```python
from build123d import *

# Parameters (mm, degrees)
F0_R     = 88.9
F1_DEPTH = 50.8
F2_R     = 60.325
F3_DEPTH = 52.07
F4_W     = 107.95
F4_H     = 63.5
F5_DEPTH = 101.6
F6_W     = 107.95
F6_H     = 63.5
F7_DEPTH = 101.6


with BuildPart() as f1:
    # F0 (on Top) → F1 (new body, symmetric)
    with BuildSketch(Plane.XY):
        Circle(F0_R)
    extrude(amount=F1_DEPTH, both=True)

    # F2 (on Top) → F3 (cut, symmetric)
    with BuildSketch(Plane.XY):
        Circle(F2_R)
    extrude(amount=F3_DEPTH, both=True, mode=Mode.SUBTRACT)

    # F4 (on Front) → F5 (cut, symmetric)
    with BuildSketch(Plane.XZ):
        Rectangle(F4_W, F4_H)
    extrude(amount=F5_DEPTH, both=True, mode=Mode.SUBTRACT)

    # F6 (on Right) → F7 (cut, symmetric)
    with BuildSketch(Plane.YZ):
        Rectangle(F6_W, F6_H)
    extrude(amount=F7_DEPTH, both=True, mode=Mode.SUBTRACT)


solid = f1.part
```
Build history of the part. All positions in model axes, mm. A direction names the side the tool comes from. Round coordinates to 2 decimals unless told otherwise and drop trailing zeros. Loops run counter-clockwise (first coordinate to the right, second up) from the corner with the lowest first, then second, coordinate; pieces in that order, holes last.
Item 1: Drill centre lines: line 1 along Y through (x, z) = (2, 47.5); line 2 along Z through (x, y) = (-80.5, -26); line 3 along X through (y, z) = (0, -39.25) (3 decimals). Where is each one in solid material? Low to high.
Item 2: Pin check, flat tips, straight feed: P1, Ø13.5, axis at y = 63, z = -12, coming from the -X side; P2, Ø13.5, axis at x = 65, z = 8.5, coming from the -Y side; P3, Ø12, axis at x = -67, z = 22.5, coming from the +Y side. Stop position of each tip, or through.
Item 3: Which spindle directions (+Z, -Z, +X, -X, +Y, -Y) get a long thin tool onto all of the face, cutting with end or side? Do faces 4 (the face through (62, -53.975, 0)), 5 (the face through (53.975, -62, 0)), 6 (the face through (-58, 19, -31.75)). Say none if no direction does.
Item 4: Two-plate mould, pull along X, no slides. Class faces 1 (the face through (-62, -53.975, 0)), 2 (the face through (-60.267, 2.652, -41.142)), 3 (the face through (-65.523, 60.083, 0.711)): released by +X, released by -X, zero draft, split by the parting line, or undercut.
Item 5: Saw through at A-A (z = -11). List the corners of the cut face in (x, y) (3 decimals), then the cut area to 3 significant figures.
Item 6: Saw through at B-B (x = 0). List the corners of the cut face in (y, z) (3 decimals).
Item 7: Saw through at D-D (z = -39.5). List the corners of the cut face in (x, y) (3 decimals).
Worked answers:
1. line 1: y = -88.88 to -60.29, 60.29 to 88.88
1. line 2: z = -50.8 to -31.75, 31.75 to 50.8
1. line 3: x = -88.9 to -60.325, 60.325 to 88.9
2. P1: stops at x = -68.84
2. P2: stops at y = -67.16
2. P3: stops at y = 64.67
3. face 4: +X, -X
3. face 5: +Y, -Y
3. face 6: none
4. face 1: zero draft
4. face 2: undercut
4. face 3: split by the parting line
5. outline: (-70.639, -53.975) arc R88.9 ccw to (-53.975, -70.639) - (-53.975, -53.975) - close; (-70.639, 53.975) - (-53.975, 53.975) - (-53.975, 70.639) arc R88.9 ccw to start; (53.975, -70.639) arc R88.9 ccw to (70.639, -53.975) - (53.975, -53.975) - close; (53.975, 53.975) - (70.639, 53.975) arc R88.9 ccw to (53.975, 70.639) - close
5. area: 605 mm2
6. outline: (-88.9, -50.8) - (-60.325, -50.8) - (-60.325, -31.75) - (-88.9, -31.75) - close; (-88.9, 31.75) - (-60.325, 31.75) - (-60.325, 50.8) - (-88.9, 50.8) - close; (60.325, -50.8) - (88.9, -50.8) - (88.9, -31.75) - (60.325, -31.75) - close; (60.325, 31.75) - (88.9, 31.75) - (88.9, 50.8) - (60.325, 50.8) - close
7. outline: circle Ø177.8 at (0, 0); hole circle Ø120.65 at (0, 0)
